Here's how the part is built. I have some questions about the finished solid (model axes, mm). Face numbers are marked on the shaded views. A direction names the side the tool comes from. Round coordinates to 2 decimals unless told otherwise and drop trailing zeros. Loops run counter-clockwise (first coordinate to the right, second up) from the corner with the lowest first, then second, coordinate; pieces in that order, holes last. Notation, with made-up numbers: M 67,-8.5 L 121,-8.5 A27 cw 121,18.5 Z; hole C -6,75.5 d11. An arc over 180 degrees is marked long. Answer as a JSON object with one key per item and string values.
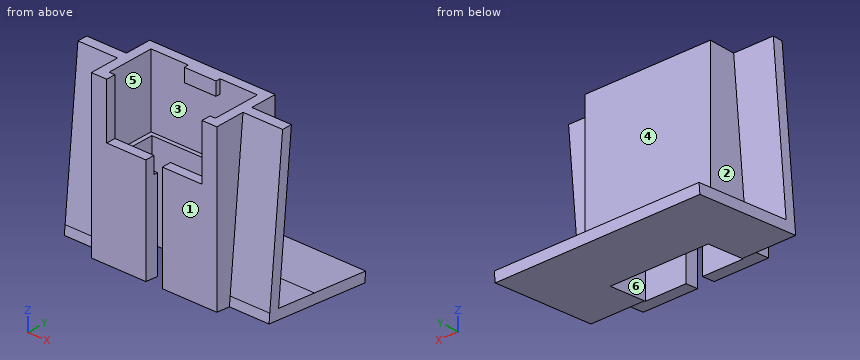
from build123d import *

# Parameters (mm, degrees)
F0_W           = 19
F0_H           = 10
F0_W_2         = 16.1
F0_H_2         = 7.2
F1_DEPTH       = 10.8
F0_W_3         = 14.7984437644
F0_H_3         = 6.0001779348
F2_DEPTH       = 12.2
F4_DEPTH       = 6
F4_DEPTH_BACK  = 25
F5_DEPTH       = 19
F6_DEPTH       = 15.1224483792
F7_DEPTH       = 25
F8_W           = 14.4229265861
F8_H           = 8.3078492425
F9_DEPTH       = 25
F10_W          = 4.8
F10_H          = 2
F11_DEPTH      = 0.7
F12_W          = 2.5
F12_H          = 5
F13_DEPTH      = 25
F13_DEPTH_BACK = 25


with BuildPart() as f1:
    # F0 (on Top) → F1 (new body)
    with BuildSketch(Plane.XY):
        Rectangle(F0_W, F0_H)
        Rectangle(F0_W_2, F0_H_2, mode=Mode.SUBTRACT)
    extrude(amount=F1_DEPTH)

    # F0 (on Top) → F2 (join)
    with BuildSketch(Plane.XY):
        Rectangle(F0_W, F0_H)
        Rectangle(F0_W_2, F0_H_2, mode=Mode.SUBTRACT)
        Rectangle(F0_W_2, F0_H_2)
        Rectangle(F0_W_3, F0_H_3, mode=Mode.SUBTRACT)
    extrude(amount=-F2_DEPTH)

    # F3 (on face) → F4 (join, two sides)
    with BuildSketch(Plane(origin=(-9.5, 0, 0), x_dir=(0, -1, 0), z_dir=(-1, 0, 0))) as f4_sk:
        Polygon((0.4931847272, 10.8), (-1, 10.8), (1.2, -12.2), (2.7068463795, -12.2), (0.5068463795, 10.8), align=None)
        Polygon((2.7068463795, -12.2), (1.2, -12.2), (-4.943788401, -12.7876667166), (-13.7318472715, -13.6282636521), (-13.5890209063, -15.1214483792), (2.8360110924, -13.5503583619), align=None)
    extrude(amount=F4_DEPTH)
    extrude(f4_sk.sketch, amount=-F4_DEPTH_BACK)

    # F3 (on face) → F5 (join)
    with BuildSketch(Plane(origin=(-9.5, 0, 0), x_dir=(0, -1, 0), z_dir=(-1, 0, 0))):
        Polygon((-4.943788401, -12.7876667166), (1.2, -12.2), (-5, -12.2), align=None)
        Polygon((5, -12.2), (2.7068463795, -12.2), (2.8360110924, -13.5503583619), (5, -13.3433681186), align=None)
    extrude(amount=-F5_DEPTH)

    # F0 (on Top) → F6 (cut, through all)
    with BuildSketch(Plane.XY):
        Rectangle(F0_W_3, F0_H_3)
    extrude(amount=-F6_DEPTH, mode=Mode.SUBTRACT)

    # F0 (on Top) → F7 (cut)
    with BuildSketch(Plane.XY):
        Rectangle(F0_W_2, F0_H_2)
        Rectangle(F0_W_3, F0_H_3, mode=Mode.SUBTRACT)
        Rectangle(F0_W_3, F0_H_3)
    extrude(amount=F7_DEPTH, mode=Mode.SUBTRACT)

    # F8 (on face) → F9 (cut)
    with BuildSketch(Plane(origin=(0, -3.6, 0), x_dir=(-1, 0, 0), z_dir=(0, 1, 0))):
        with Locations((-0.0403469894, 6.6460753787)):
            Rectangle(F8_W, F8_H)
    extrude(amount=-F9_DEPTH, mode=Mode.SUBTRACT)

    # F10 (on face) → F11 (join)
    with BuildSketch(Plane.XZ.offset(-3.6)):
        with Locations((0, 9.8)):
            Rectangle(F10_W, F10_H)
    extrude(amount=F11_DEPTH)

    # F12 (on Top) → F13 (cut, two sides)
    with BuildSketch(Plane.XY) as f13_sk:
        with Locations((0, -4.9948594533)):
            Rectangle(F12_W, F12_H)
    extrude(amount=-F13_DEPTH, mode=Mode.SUBTRACT)
    extrude(f13_sk.sketch, amount=F13_DEPTH_BACK, mode=Mode.SUBTRACT)


solid = f1.part
Item 1: I want a section at D-D, the plane z = 8. Please give me the cut outline in (x, y).
Resolved:
{"outline": "M -15.5,-0.77 L -9.5,-0.77 L -9.5,-5 L -7.17,-5 L -7.17,-3.6 L -8.05,-3.6 L -8.05,3.6 L 8.05,3.6 L 8.05,-3.6 L 7.25,-3.6 L 7.25,-5 L 9.5,-5 L 9.5,-0.77 L 15.5,-0.77 L 15.5,0.73 L 9.5,0.73 L 9.5,5 L -9.5,5 L -9.5,0.73 L -15.5,0.73 Z"}
Item 2: I want a section at C-C, the plane x = 11. Please give me the cut outline in (y, z).
Resolved:
{"outline": "M -2.84,-13.55 L 13.59,-15.12 L 13.73,-13.63 L -1.2,-12.2 L 1,10.8 L -0.51,10.8 Z"}
Item 3: I'm going to push flat-ended pins straight in: pin 1 Ø8 at (x, y) = (0, 6.5) entering from -Z; pin 2 Ø1.5 at (y, z) = (-4, 7) entering from +X; pin 3 Ø0.7 at (y, z) = (-4, 6.5) entering from -X. Where does each tip first touch, or does it pass through?
Resolved:
{"pin 1": "z = -14.83", "pin 2": "x = 9.5", "pin 3": "x = -9.5"}
Item 4: On a 3-axis mill with a long thin cutter (end or side, diameter ignored), from which of +Z, -Z, +X, -X, +Y, -Y can I reach the whole of each face in a straight line? I mean the marked faces 4, 5 and 6. Say none if no direction works.
Resolved:
{"face 4": "+Z, +X, -X, +Y", "face 5": "+Z", "face 6": "+Z, -Z"}
Item 5: I want a section at B-B, the plane y = 2. Please give me the cut outline in (x, z), then the cut area to 3 significant figures.
Resolved:
{"outline": "M -15.5,-14.01 L -7.4,-14.01 L -7.4,0 L -8.05,0 L -8.05,10.8 L -9.5,10.8 L -9.5,-12.51 L -15.5,-12.51 Z; M 7.4,-14.01 L 15.5,-14.01 L 15.5,-12.51 L 9.5,-12.51 L 9.5,10.8 L 8.05,10.8 L 8.05,0 L 7.4,0 Z", "area": "108 mm²"}
Item 6: I want a section at A-A, the plane x = -6. Please give me the cut outline in (y, z), then the cut area to 3 significant figures.
Resolved:
{"outline": "M -5,-13.34 L -3,-13.53 L -3,0 L -3.6,0 L -3.6,2.49 L -5,2.49 Z; M 3,-14.11 L 13.59,-15.12 L 13.73,-13.63 L 4.94,-12.79 L 5,-12.2 L 5,10.8 L 3.6,10.8 L 3.6,0 L 3,0 Z", "area": "86.9 mm²"}
Item 7: Please list where these lines run through material, in increasing order: probe 1 along X at (y, z) = (-3, 3.5); probe 2 along X at (y, z) = (-3.5, -10.5); probe 3 along Y at (x, z) = (-6, -9). Write a range as from..to.
Resolved:
{"probe 1": "-9.5..-8.05, 8.05..9.5", "probe 2": "-9.5..-1.25, 1.25..9.5", "probe 3": "-5..-3, 3..5"}
Item 8: If we mould it in two halves opening along X, with no side actions, what happens to the marked faces 1, 2 and 3? For each: pulls with the +X half, pulls with the -X half, needs draft (parallel to the pull), parting line crosses it, or undercut.
Resolved:
{"face 1": "needs draft", "face 2": "pulls with the -X half", "face 3": "undercut"}
